Answer from the drawing. Dimensions are ordinates in mm from the lowest x, y and z of the part. Give positions to 0.01 mm unless a question says otherwise; leave off trailing zeros. Write each loop counter-clockwise with the first axis right and the second up, starting at its lowest first coordinate (ties: lowest second). Pieces come first, ordered by that corner, then holes. Notation, with made-up numbers: (8, -36.75) -> (64, -36.75) arc R16 cw to (64, -32.75) -> close; hole circle Ø9 at (46, -7). An arc over 180 degrees is marked (long way). Put each result on its own line as item: value. Start each with the question number.
1) Find the intervals of material crossed by line 1 along Z through (x, y) = (25.5, 1.25) (1 decimal); line 2 along X through (y, z) = (1, 4); line 3 along X through (y, z) = (2.9, 19) (1 decimal), in increasing order. Write a range as from..to.
2) A cutting plane is placed at A-A (x = 17.78). Write down the section's boundary in (y, z) (1 decimal).
3) A cutting plane is placed at B-B (z = 12.7). Write down the section's boundary in (x, y) (1 decimal).
4) A cutting plane is placed at D-D (z = 7.75). Write down the section's boundary in (x, y) (1 decimal).
5) A cutting plane is placed at C-C (x = 24). Write down the section's boundary in (y, z) (1 decimal).
6) For a pull along X with two mould halves and no side action, classify the marked faces 1 and 2 as released by +X, released by -X, zero draft, split by the parting line, or undercut.
7) Flat-ended cylindrical pins translate along their axes: pin 1 Ø2 at (x, z) = (24.38, 17.73) entering from -Y; pin 2 Ø1 at (x, z) = (5.5, 3.5) entering from -Y. Find the tip coordinate at first contact, or state that the pin passes through.
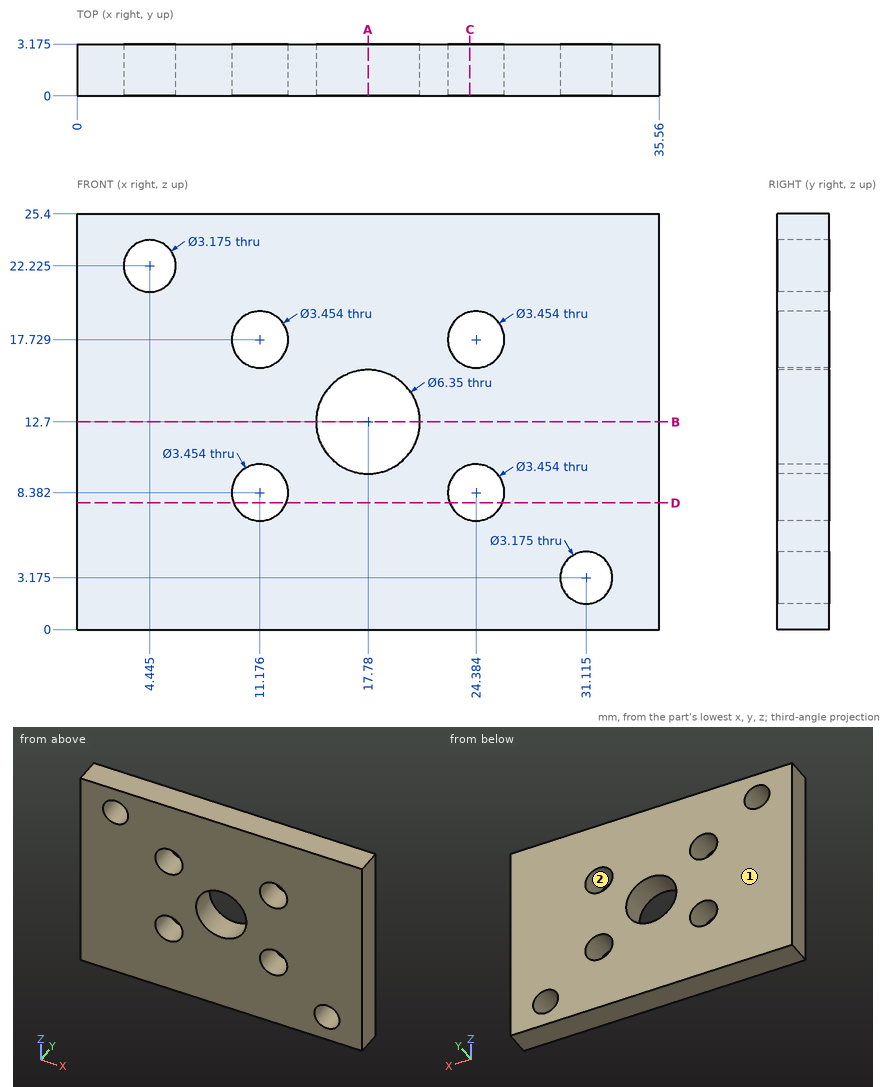
Reply:
1. line 1: z = 0..7.1, 9.7..16.4, 19..25.4
1. line 2: x = 0..29.76, 32.47..35.56
1. line 3: x = 0..10, 12.3..23.2, 25.6..35.6
2. outline: (0, 0) -> (3.2, 0) -> (3.2, 9.5) -> (0, 9.5) -> close; (0, 15.9) -> (3.2, 15.9) -> (3.2, 25.4) -> (0, 25.4) -> close
3. outline: (0, 0) -> (14.6, 0) -> (14.6, 3.2) -> (0, 3.2) -> close; (21, 0) -> (35.6, 0) -> (35.6, 3.2) -> (21, 3.2) -> close
4. outline: (0, 0) -> (9.6, 0) -> (9.6, 3.2) -> (0, 3.2) -> close; (12.8, 0) -> (22.8, 0) -> (22.8, 3.2) -> (12.8, 3.2) -> close; (26, 0) -> (35.6, 0) -> (35.6, 3.2) -> (26, 3.2) -> close
5. outline: (0, 0) -> (3.2, 0) -> (3.2, 6.7) -> (0, 6.7) -> close; (0, 10.1) -> (3.2, 10.1) -> (3.2, 16) -> (0, 16) -> close; (0, 19.4) -> (3.2, 19.4) -> (3.2, 25.4) -> (0, 25.4) -> close
6. face 1: zero draft
6. face 2: undercut
7. pin 1: passes through
7. pin 2: stops at y = 0
